```python
from build123d import *

# Parameters (mm, degrees)
F1_DEPTH = 41.275
F2_R     = 4.7625
F3_DEPTH = 88.901
F4_R     = 6.35
F4_R_2   = 4.7625
F5_DEPTH = 101.601


with BuildPart() as f1:
    # F0 (on Top) → F1 (new body, symmetric)
    with BuildSketch(Plane.XY):
        Polygon((-82.55, 0), (0, 0), (0, -95.25), (6.35, -95.25), (6.35, 6.35), (-82.55, 6.35), align=None)
    extrude(amount=F1_DEPTH, both=True)

    # F2 (on face) → F3 (cut, through all)
    with BuildSketch(Plane.YZ.offset(6.35)):
        with Locations((-69.85, 17.4625)):
            Circle(F2_R)
        with Locations((-69.85, -17.4625)):
            Circle(F2_R)
    extrude(amount=-F3_DEPTH, mode=Mode.SUBTRACT)

    # F4 (on face) → F5 (cut, through all)
    with BuildSketch(Plane(origin=(0, 6.35, 0), x_dir=(-1, 0, 0), z_dir=(0, 1, 0))):
        with Locations((63.5, 13.4874)):
            Circle(F4_R)
        with Locations((63.5, -13.4874)):
            Circle(F4_R)
        with Locations((19.05, 0)):
            Circle(F4_R_2)
    extrude(amount=-F5_DEPTH, mode=Mode.SUBTRACT)


solid = f1.part
```
Source: CAD feature listing. Evaluate the final solid. Frame: model axes, mm. A direction names the side the tool comes from. Give positions to 0.01 mm unless a question says otherwise; leave off trailing zeros. Loops run counter-clockwise (first coordinate to the right, second up) from the corner with the lowest first, then second, coordinate; pieces in that order, holes last. Notation, with made-up numbers: (25.25, 54) -> (67.25, 54) arc R16 ccw to (67.25, 70) -> close; hole circle Ø10 at (-35.5, 85.25). An arc over 180 degrees is marked (long way). Use a Markdown table: item, result. Add a question column.
(1) First-contact query: pin 1 Ø6 at (x, z) = (-38, 12.5) entering from -Y; pin 2 Ø12.5 at (y, z) = (-69.85, -17.46) entering from -X. Flat tips, straight axial feed; report the tip coordinate or a pass-through.
(2) Pull-direction query (X, two-part tool) for faces 1 (the face through (-66.91, 3.22, -8.13)), 2 (the face through (-82.55, 3, 1)), 3 (the face through (1, -22, -41.275)); classes: +X half, -X half, draft (parallel to the pull), parting line (faces both ways), or undercut.
(3) Section query C-C (x = -63.5). Output: boundary loops of the cut face in (y, z) (3 decimals).
(4) Section query B-B (z = 0). Output: boundary loops of the cut face in (x, y).
(5) Ray query, line 1 (Z direction, x = 2, y = -69.85) (3 decimals); line 2 (Z direction, x = -19.05, y = 1.5) (1 decimal); line 3 (Z direction, x = 5, y = -69) (3 decimals). Return the intervals inside material, ascending.
(6) Access query for faces 4 (the face through (0, -47, 1)), 5 (the face through (-14.292, 3.219, 0.209)). Directions: +Z, -Z, +X, -X, +Y, -Y. A direction counts if a zero-diameter tool reaches every point of the face in a straight line with its end or side. Return the directions, or none.
(7) Section query D-D (y = -52.5). Output: boundary loops of the cut face in (x, z) (3 decimals).
Checked values:
| question | item | result |
|---|---|---|
| 1 | pin 1 | y = 0 |
| 1 | pin 2 | x = 0 |
| 2 | face 1 | undercut |
| 2 | face 2 | -X half |
| 2 | face 3 | draft |
| 3 | outline | (0, -41.275) -> (6.35, -41.275) -> (6.35, -19.837) -> (0, -19.837) -> close; (0, -7.137) -> (6.35, -7.137) -> (6.35, 7.137) -> (0, 7.137) -> close; (0, 19.837) -> (6.35, 19.837) -> (6.35, 41.275) -> (0, 41.275) -> close |
| 4 | outline | (-82.55, 0) -> (-23.81, 0) -> (-23.81, 6.35) -> (-82.55, 6.35) -> close; (-14.29, 0) -> (0, 0) -> (0, -95.25) -> (6.35, -95.25) -> (6.35, 6.35) -> (-14.29, 6.35) -> close |
| 5 | line 1 | -41.275 to -22.225, -12.7 to 12.7, 22.225 to 41.275 |
| 5 | line 2 | -41.3 to -4.8, 4.8 to 41.3 |
| 5 | line 3 | -41.275 to -22.149, -12.776 to 12.776, 22.149 to 41.275 |
| 6 | face 4 | +Z, -Z, -X, -Y |
| 6 | face 5 | +Y, -Y |
| 7 | outline | (0, -41.275) -> (6.35, -41.275) -> (6.35, 41.275) -> (0, 41.275) -> close |
